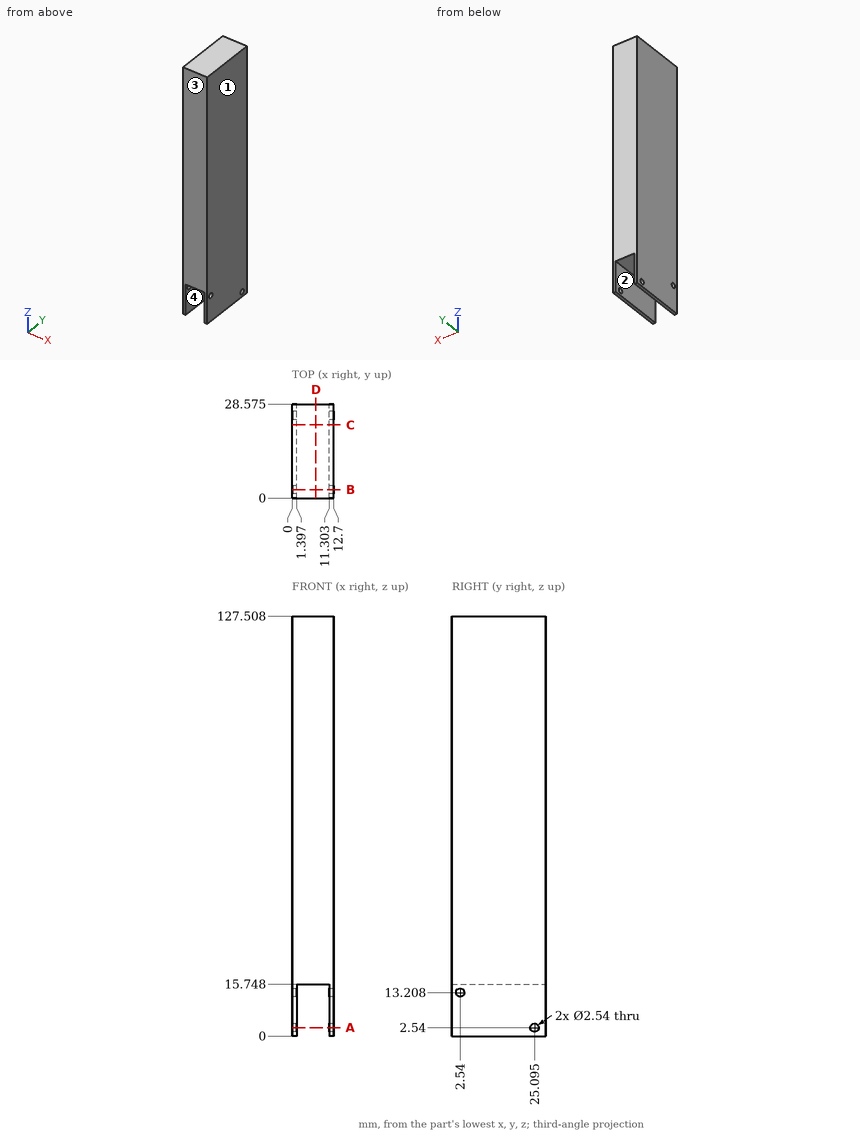
Verification items for this drawing (mm, ordinates from the low corner). Give positions to 0.01 mm unless a question says otherwise; leave off trailing zeros. Write each loop counter-clockwise with the first axis right and the second up, starting at its lowest first coordinate (ties: lowest second). Pieces come first, ordered by that corner, then holes.
1) Gauge pin test, flat end, axial feed: pin 1 (3 mm diameter, centred on x = 5.5, y = 9, fed in from -Z). Record the tip position at first contact, or that the pin passes through.
2) Section check A-A, the plane z = 2.54. Record the boundary of the cut face in (x, y) (1 decimal).
3) Material ranges on L1, parallel to Y at x = 11.85, z = 2.54 (1 decimal); L2, parallel to Z at x = 2, y = 24.25, recorded low to high.
4) Release check for a two-part mould opening along X. For the marked faces 1, 2, 3 and 4 record: pulls with the +X half, pulls with the -X half, needs draft (parallel to the pull), parting line crosses it, or undercut.
5) Section check D-D, the plane x = 7.25. Record the boundary of the cut face in (y, z) (3 decimals), and give its area (3 significant figures).
6) Section check C-C, the plane y = 22.25. Record the boundary of the cut face in (x, z).
7) Section check B-B, the plane y = 2.54. Record the boundary of the cut face in (x, z), and give its area (3 significant figures).
Computed:
1. pin 1: stops at z = 15.75
2. outline: (0, 0) - (1.4, 0) - (1.4, 23.8) - (0, 23.8) - close; (0, 26.4) - (1.4, 26.4) - (1.4, 28.6) - (0, 28.6) - close; (11.3, 0) - (12.7, 0) - (12.7, 23.8) - (11.3, 23.8) - close; (11.3, 26.4) - (12.7, 26.4) - (12.7, 28.6) - (11.3, 28.6) - close
3. L1: y = 0 to 23.8, 26.4 to 28.6
3. L2: z = 15.75 to 127.51
4. face 1: pulls with the +X half
4. face 2: undercut
4. face 3: needs draft
4. face 4: undercut
5. outline: (0, 15.748) - (28.575, 15.748) - (28.575, 127.508) - (0, 127.508) - close
5. area: 3,190 mm2
6. outline: (0, 0) - (1.4, 0) - (1.4, 15.75) - (11.3, 15.75) - (11.3, 0) - (12.7, 0) - (12.7, 127.51) - (0, 127.51) - close
7. outline: (0, 0) - (1.4, 0) - (1.4, 11.94) - (0, 11.94) - close; (0, 14.48) - (1.4, 14.48) - (1.4, 15.75) - (11.3, 15.75) - (11.3, 14.48) - (12.7, 14.48) - (12.7, 127.51) - (0, 127.51) - close; (11.3, 0) - (12.7, 0) - (12.7, 11.94) - (11.3, 11.94) - close
7. area: 1,460 mm2
